Geometry check sheet. Reference: drawing and pictorial views, mm from the part's lowest x, y, z. Round coordinates to 2 decimals unless told otherwise and drop trailing zeros. Loops run counter-clockwise (first coordinate to the right, second up) from the corner with the lowest first, then second, coordinate; pieces in that order, holes last. Notation, with made-up numbers: (88, 1.25) - (145, 1.25) arc R8 cw to (145, 14.25) - close; hole circle Ø2 at (11.5, 67). An arc over 180 degrees is marked (long way). Answer as CSV lines item,"result". Start each with the question number.
1) Depth check by flat-ended pin: P1, Ø1, axis at y = 14.5, z = 4.5, coming from the +X side; P2, Ø5, axis at x = 12.5, z = 2, coming from the +Y side; P3, Ø6, axis at x = 41, y = 35.5, coming from the -Z side; P4, Ø4, axis at x = 29.5, y = 29.5, coming from the +Z side. Enter the tip coordinate at first touch or a pass-through.
2) Thickness scan on line 1 along Y through (x, z) = (29.5, 12.5); line 2 along Z through (x, y) = (24.5, 27); line 3 along Y through (x, z) = (41.5, 10.5). Record the ranges inside material, lowest first.
3) Draft check along X on the marked faces 1, 2 and 3. Enter one of: released by +X, released by -X, zero draft, split by the parting line, or undercut.
4) Cross-section at D-D on y = 5. Record the boundary of the cut face in (x, z), and give its area (3 significant figures).
5) Cross-section at B-B on y = 29.5. Record the boundary of the cut face in (x, z).
6) Cross-section at A-A on x = 29.5. Record the boundary of the cut face in (y, z).
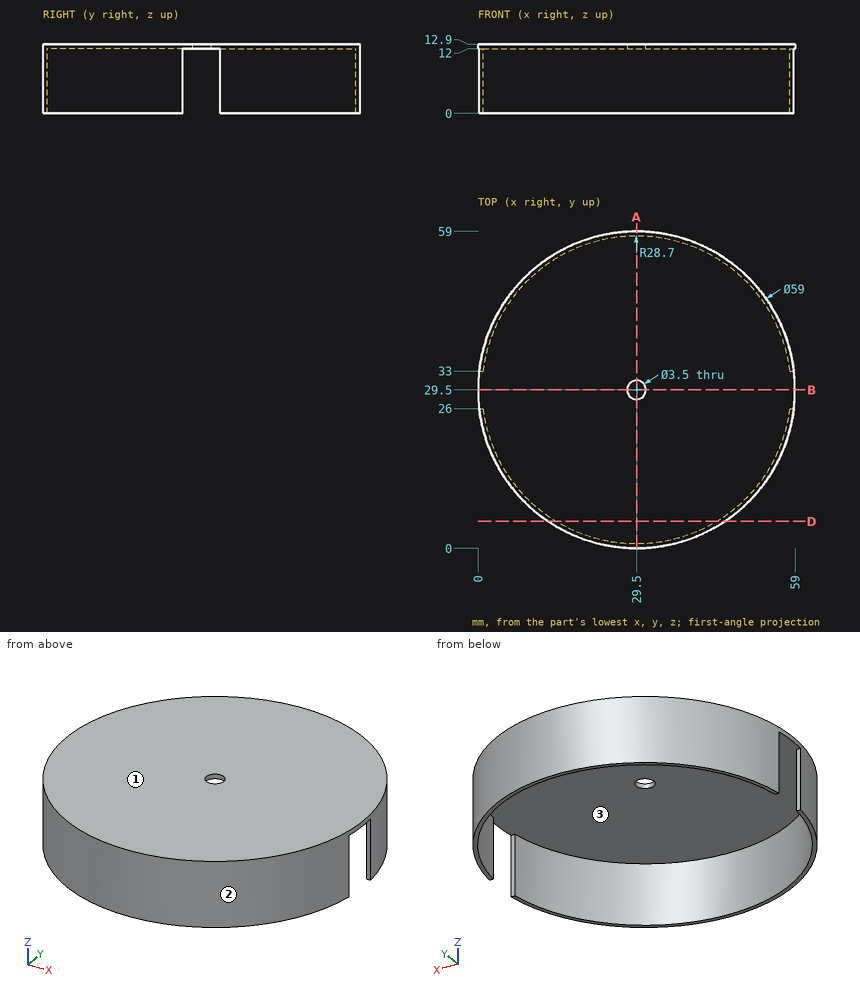
Answer block:
1,P1,"stops at x = 55.19"
1,P2,"stops at y = 55.19"
1,P3,"stops at z = 12"
1,P4,"stops at z = 12.9"
2,line 1,"y = 0 to 27.75, 31.25 to 59"
2,line 2,"z = 12 to 12.9"
2,line 3,"y = 2.55 to 3.43, 55.57 to 56.45"
3,face 1,"zero draft"
3,face 2,"split by the parting line"
3,face 3,"undercut"
4,outline,"(13.07, 0) - (14.55, 0) - (14.55, 12) - (44.45, 12) - (44.45, 0) - (45.93, 0) - (45.93, 12.9) - (13.07, 12.9) - close"
4,area,"65.2 mm^2"
5,outline,"(0, 12) - (27.75, 12) - (27.75, 12.9) - (0, 12.9) - close; (31.25, 12) - (59, 12) - (59, 12.9) - (31.25, 12.9) - close"
6,outline,"(0, 0) - (0.8, 0) - (0.8, 12) - (27.75, 12) - (27.75, 12.9) - (0, 12.9) - close; (31.25, 12) - (58.2, 12) - (58.2, 0) - (59, 0) - (59, 12.9) - (31.25, 12.9) - close"
